from build123d import *

# Parameters (mm, degrees)
BOSS_EXTRUDE2_DEPTH = 1.37
FILLET1_R           = 2
CUT_EXTRUDE1_REACH  = 88.37
SKETCH3_R           = 7.2


with BuildPart() as part:
    # Sketch1 → Revolve1 (revolve)
    with BuildSketch(Plane.XY):
        Polygon((8.3, 86.37), (8.2, 10.576282817), (4.71, 8.87), (4.71, 0), (3.96, 0), (3.96, 4.391129032), (2, 4.391129032), (2, 0), (1, 0), (1, 8.169274748), (7.2, 11.200493506), (7.2, 86.37), align=None)
    revolve(axis=Axis((0, 0, 0), (0, 1, 0)))

    # Sketch2 → Boss-Extrude2 (add)
    with BuildSketch(Plane(origin=(0, 86.37, 0), x_dir=(1, 0, 0), z_dir=(0, 1, 0))):
        with BuildLine():
            Line((2.056176332, 9.274812068), (13.180263935, 6.808661219))
            ThreePointArc((13.180263935, 6.808661219), (14.835, 0), (13.180263935, -6.808661219))
            Line((13.180263935, -6.808661219), (2.056176332, -9.274812068))
            ThreePointArc((2.056176332, -9.274812068), (0, -9.5), (-2.056176332, -9.274812068))
            Line((-2.056176332, -9.274812068), (-13.180263935, -6.808661219))
            ThreePointArc((-13.180263935, -6.808661219), (-14.835, 0), (-13.180263935, 6.808661219))
            Line((-13.180263935, 6.808661219), (-2.056176332, 9.274812068))
            ThreePointArc((-2.056176332, 9.274812068), (0, 9.5), (2.056176332, 9.274812068))
        make_face()
    extrude(amount=-BOSS_EXTRUDE2_DEPTH)

    # Fillet1
    fillet1_edges = [part.edges().sort_by_distance(p)[0] for p in [
        (13.180263935, 85.685, -6.808661219),
        (13.180263935, 85.685, 6.808661219),
        (-13.180263935, 85.685, 6.808661219),
        (-13.180263935, 85.685, -6.808661219),
    ]]
    fillet(fillet1_edges, radius=FILLET1_R)

    # Sketch3 → Cut-Extrude1 (cut, up to next)
    with BuildSketch(Plane(origin=(0, 86.37, 0), x_dir=(1, 0, 0), z_dir=(0, 1, 0)), mode=Mode.PRIVATE) as cut_extrude1_sk1:
        Circle(SKETCH3_R)
    cut_extrude1_tool1 = extrude(cut_extrude1_sk1.sketch, amount=-CUT_EXTRUDE1_REACH, mode=Mode.PRIVATE) & part.part
    add(cut_extrude1_tool1.solids().sort_by_distance((0, 86.37, 0))[0], mode=Mode.SUBTRACT)


solid = part.part
Verification items for the finished model (mm, model axes). A direction names the side the tool comes from. Coordinates: 2 decimals unless noted, no trailing zeros. Loops run counter-clockwise (first coordinate to the right, second up) from the corner with the lowest first, then second, coordinate; pieces in that order, holes last. Notation, with made-up numbers: M 50,61.5 L 56,61.5 A28 ccw 56,86.5 Z; hole C 19,35 d5. An arc over 180 degrees is marked long. One line per item, written item: value.
1. Set-up check for faces 5 (the cylindrical face through (6.87, 49.31, -2.16)), 6 (the flat face through (-6, 85, 6)), 7 (the flat face through (-1, 0, -4)): record each of +Z, -Z, +X, -X, +Y, -Y from which the full face is reachable in a straight line by a thin tool's end or side.
Answers follow:
face 5: +Y
face 6: -Y
face 7: +Z, -Z, +X, -X, -Y
2. Mould release check, pull along Z, two halves, no side actions. Record for faces 1 (the flat face through (-7.212, 85.695, -8.132)), 2 (the flat face through (1, 0, 1)), 3 (the conical face through (-2, 47, 8)), 4 (the flat face through (-2, 4.391, -1)): pulls with the +Z half, pulls with the -Z half, needs draft (parallel to the pull), parting line crosses it, or undercut.
Answers follow:
face 1: pulls with the -Z half
face 2: needs draft
face 3: parting line crosses it
face 4: undercut
3. Section check A-A on y = 41. Record the cut outline in (x, z), plus the area to 3 significant figures.
Answers follow:
outline: C 0,0 d16.48; hole C 0,0 d14.4
area: 50.5 mm^2
4. Section check B-B on y = 22. Record the cut outline in (x, z), plus the area to 3 significant figures.
Answers follow:
outline: C 0,0 d16.43; hole C 0,0 d14.4
area: 49.2 mm^2
5. Material ranges on line 1 along X through (y, z) = (4.25, 0); line 2 along X through (y, z) = (4.75, 0), recorded low to high. Write a range as from..to.
Answers follow:
line 1: -4.71..-3.96, -2..-1, 1..2, 3.96..4.71
line 2: -4.71..-1, 1..4.71
6. Gauge pin test, flat ends, axial feed: P1, Ø8, axis at x = 5.5, y = 47.5, coming from the +Z side; P2, Ø8.5, axis at x = 1, z = 0.5, coming from the -Y side; P3, Ø4, axis at x = 0, y = 27, coming from the -Z side; P4, Ø10.5, axis at x = 0, z = 0, coming from the +Y side. Record the tip position at first contact, or that the pin passes through.
Answers follow:
P1: z = 8.11
P2: y = 0
P3: z = -8.22
P4: y = 10.25
